Work out the finished part from the listing and answer in its coordinate system (mm). A direction names the side the tool comes from. Round coordinates to 2 decimals unless told otherwise and drop trailing zeros. Write each loop counter-clockwise with the first axis right and the second up, starting at its lowest first coordinate (ties: lowest second). Pieces come first, ordered by that corner, then holes. Notation, with made-up numbers: (11.25, 79.5) - (39.25, 79.5) arc R11 cw to (39.25, 91.5) - close; hole circle Ø9 at (71.25, 7.25). An arc over 180 degrees is marked (long way). Write item = value, one per line. Start each with the question number.
Autodesk Inventor part; units mm, degrees
ref_plane "YZ Plane" through (0, 0, 0) normal (1, 0, 0) x (0, 1, 0)
ref_plane "XZ Plane" through (0, 0, 0) normal (0, 1, 0) x (-1, 0, 0)
ref_plane "XY Plane" through (0, 0, 0) normal (0, 0, 1) x (1, 0, 0)
sketch "Sketch1" plane through (0, 0, 0) normal (0, 1, 0) x (-1, 0, 0)
  line L0 (-100, 10) -> (100, 10)
  line L1 (100, 10) -> (100, -10)
  line L2 (100, -10) -> (-100, -10)
  line L3 (-100, -10) -> (-100, 10)
  line L4 (-100, 10) -> (100, -10) construction
  line L5 (100, 10) -> (-100, -10) construction
  point P0 (0, 0)
  dimension "d0" = 200
  dimension "d1" = 20
extrude "Extrusion1" add sketch "Sketch1" along normal blind 5
sketch "Sketch2" plane through (0, 5, 0) normal (0, 1, 0) x (1, 0, 0)
  line L0 (97.5, 2.5) -> (102.5, 2.5)
  line L1 (102.5, 2.5) -> (102.5, -2.5)
  line L2 (102.5, -2.5) -> (97.5, -2.5)
  line L3 (97.5, -2.5) -> (97.5, 2.5)
  line L4 (100, -10) -> (100, 10)
  line L5 (97.5, 2.5) -> (102.5, -2.5) construction
  line L6 (102.5, 2.5) -> (97.5, -2.5) construction
  line L7 (97.5, -2.5) -> (97.5, -10)
  line L8 (-100, -10) -> (100, -10)
  line L9 (97.5, -10) -> (100, -10)
  line L10 (100, -10) -> (100, 10)
  line L11 (100, 10) -> (-100, 10)
  line L12 (97.5, 10) -> (97.5, 2.5)
  point P0 (0, 0)
  point P1 (100, 0)
  point P2 (100, 2.5)
  point P3 (100, -2.5)
  dimension "d4" = 5
  dimension "d5" = 5
extrude "Extrusion2" cut sketch "Sketch2" against normal blind 5 contours L12 L11 L4 L0 | L2 L4 L8 L7
sketch "Sketch3" plane through (0, 5, 0) normal (0, 1, 0) x (1, 0, 0)
  circle A0 centre (91.5, 0) radius 5
  line L0 (97.5, -10) -> (97.5, -2.5)
  point P0 (0, 0)
  dimension "d8" = 10
  dimension "d9" = 6
extrude "Extrusion3" cut sketch "Sketch3" against normal blind 5
properties part number "Zaxix" material "Wood (Birch)"
1. Consider line 1 (Z direction, x = 91.5, y = 1.85); line 2 (X direction, y = 2, z = 0.5); line 3 (X direction, y = 2.2, z = -7.5). Determine where each line is inside the solid, lowest interval first.
2. Which of the six approach directions +Z, -Z, +X, -X, +Y, -Y give full straight-line access (tool end or side, diameter ignored) to faces 1 (the face through (100, 2, 0)), 2 (the face through (97.5, 3, 6))?
3. Find section B-B on x = 91.5. Give the vertices of the cut face in (y, z), plus the area to 3 significant figures.
4. Find section A-A on z = 0. Give the vertices of the cut face in (x, y), plus the area to 3 significant figures.
5. For a pull along X with two mould halves and no side action, classify faces 3 (the face through (-3, 2, -10)), 4 (the face through (96.119, 2.535, 1.915)), 5 (the face through (97.5, 3, -6)) as released by +X, released by -X, zero draft, split by the parting line, or undercut.
6. Find section C-C on y = 1.85. Give the vertices of the cut face in (x, z).
7. Each of these flat-tipped pins is pushed along its axis until it touches: pin 1 (2 mm diameter, centred on x = -10, z = 0, fed in from -Y); pin 2 (1.2 mm diameter, centred on x = 98.5, y = 3, fed in from +Z). Where does it stop, or does it pass through?
Answer key:
q1.line_1 = -10 to -5, 5 to 10
q1.line_2 = -100 to 86.53, 96.47 to 100
q1.line_3 = -100 to 97.5
q2.face_1 = +Z, -Z, +X, +Y, -Y
q2.face_2 = +Z, +X, +Y, -Y
q3.outline = (0, -10) - (5, -10) - (5, -5) - (0, -5) - close; (0, 5) - (5, 5) - (5, 10) - (0, 10) - close
q3.area = 50.0 mm²
q4.outline = (-100, 0) - (86.5, 0) - (86.5, 5) - (-100, 5) - close; (96.5, 0) - (100, 0) - (100, 5) - (96.5, 5) - close
q4.area = 950 mm²
q5.face_3 = zero draft
q5.face_4 = undercut
q5.face_5 = released by +X
q6.outline = (-100, -10) - (97.5, -10) - (97.5, -2.5) - (100, -2.5) - (100, 2.5) - (97.5, 2.5) - (97.5, 10) - (-100, 10) - close; hole circle Ø10 at (91.5, 0)
q7.pin_1 = 0
q7.pin_2 = 2.5
